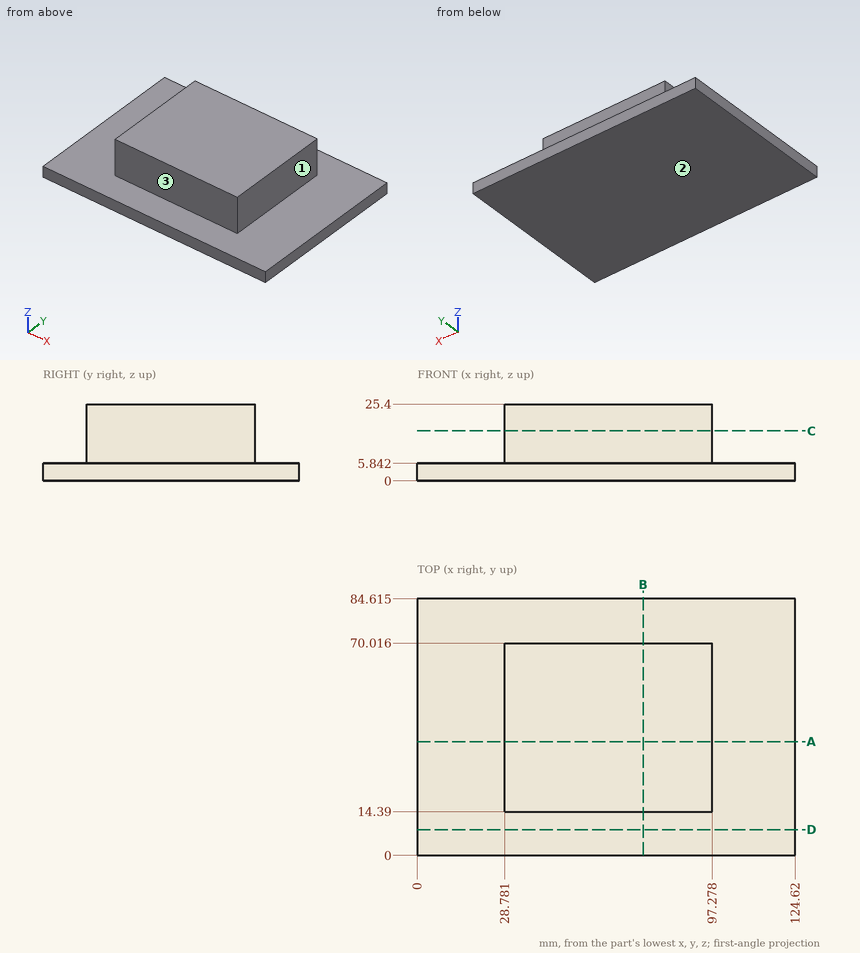
Check sheet for the drawn part. Datum: minimum x, y, z corner. Units: mm. A direction names the side the tool comes from. Round coordinates to 2 decimals unless told otherwise and drop trailing zeros. Order: outer loops, then holes, each group sorted by start corner. A loop starts at its lowest first (then second) coordinate and runs counter-clockwise, first axis right, second up. Notation, with made-up numbers: (32.25, 57.25) -> (82.25, 57.25) arc R19 cw to (82.25, 61.25) -> close; hole circle Ø2 at (12.25, 45.5). An arc over 180 degrees is marked (long way). Return JSON: item names as keys, results as strings. Group by question number.
Q1. Material ranges on probe 1 along Z at (x, y) = (111.5, 69.5); probe 2 along Y at (x, z) = (37.5, 19); probe 3 along X at (y, z) = (52, 12), recorded low to high. Write a range as from..to.
Q2. Section check B-B, the plane x = 74.5. Record the boundary of the cut face in (y, z) (1 decimal), plus the area to 3 significant figures.
Q3. Gauge pin test, flat ends, axial feed: pin 1 (6 mm diameter, centred on x = 57.5, z = 13, fed in from -Y); pin 2 (8 mm diameter, centred on y = 64, z = 15, fed in from -X); pin 3 (6 mm diameter, centred on x = 46.5, z = 12, fed in from +Y); pin 4 (3 mm diameter, centred on x = 25, y = 33, fed in from -Z). Record the tip position at first contact, or that the pin passes through.
Q4. Section check A-A, the plane y = 37.5. Record the boundary of the cut face in (x, z).
Q5. Tool access check on the marked faces 1, 2 and 3. Record the directions out of +Z, -Z, +X, -X, +Y, -Y that give a thin tool (end or side, any length) a straight path to the whole face; none if there is none.
Q6. Section check D-D, the plane y = 8.5. Record the boundary of the cut face in (x, z).
Q7. Section check C-C, the plane z = 16.5. Record the boundary of the cut face in (x, y).
Numbers:
{
 "1": {"probe 1": "0..5.84", "probe 2": "14.39..70.02", "probe 3": "28.78..97.28"},
 "2": {"outline": "(0, 0) -> (84.6, 0) -> (84.6, 5.8) -> (70, 5.8) -> (70, 25.4) -> (14.4, 25.4) -> (14.4, 5.8) -> (0, 5.8) -> close", "area": "1,580 mm^2"},
 "3": {"pin 1": "y = 14.39", "pin 2": "x = 28.78", "pin 3": "y = 70.02", "pin 4": "z = 0"},
 "4": {"outline": "(0, 0) -> (124.62, 0) -> (124.62, 5.84) -> (97.28, 5.84) -> (97.28, 25.4) -> (28.78, 25.4) -> (28.78, 5.84) -> (0, 5.84) -> close"},
 "5": {"face 1": "+Z, +X, +Y, -Y", "face 2": "-Z, +X, -X, +Y, -Y", "face 3": "+Z, +X, -X, -Y"},
 "6": {"outline": "(0, 0) -> (124.62, 0) -> (124.62, 5.84) -> (0, 5.84) -> close"},
 "7": {"outline": "(28.78, 14.39) -> (97.28, 14.39) -> (97.28, 70.02) -> (28.78, 70.02) -> close"}
}
